Source: three-view drawing plus pictorial views. Frame: mm from the lowest corner of the part. Give positions to 0.01 mm unless a question says otherwise; leave off trailing zeros. Order: outer loops, then holes, each group sorted by start corner. A loop starts at its lowest first (then second) coordinate and runs counter-clockwise, first axis right, second up. Notation, with made-up numbers: (56, 33.5) -> (91, 33.5) arc R18 cw to (91, 62.5) -> close; hole circle Ø8 at (52, 39.25). An arc over 180 degrees is marked (long way). Answer in a Markdown table with one row per item.
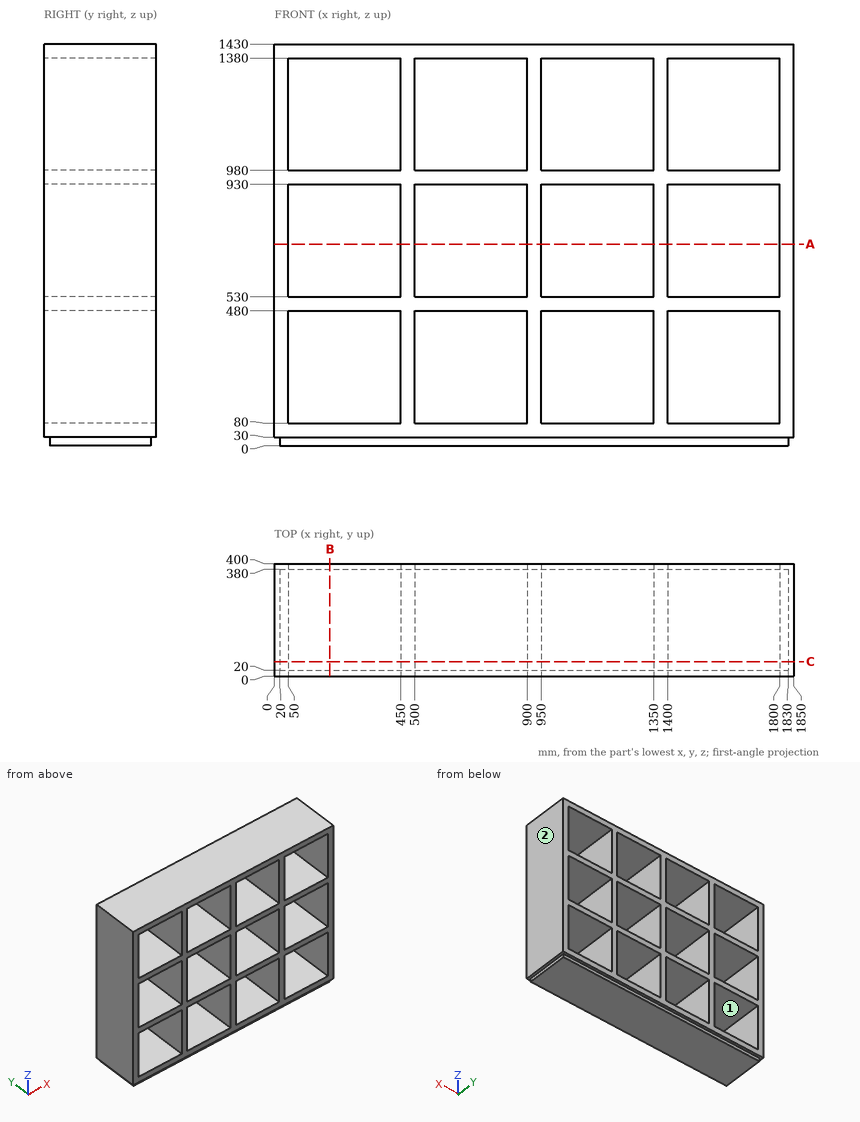
(1) Ray query, probe 1 along X at (y, z) = (269.5, 606); probe 2 along Z at (x, y) = (1578.5, 344). Return the intervals inside material, ascending.
A:
| item | result |
|---|---|
| probe 1 | x = 0 to 50, 450 to 500, 900 to 950, 1350 to 1400, 1800 to 1850 |
| probe 2 | z = 0 to 80, 480 to 530, 930 to 980, 1380 to 1430 |
(2) Section query A-A (z = 717.5). Return the cut outline in (x, y).
A:
| item | result |
|---|---|
| outline | (0, 0) -> (50, 0) -> (50, 400) -> (0, 400) -> close; (450, 0) -> (500, 0) -> (500, 400) -> (450, 400) -> close; (900, 0) -> (950, 0) -> (950, 400) -> (900, 400) -> close; (1350, 0) -> (1400, 0) -> (1400, 400) -> (1350, 400) -> close; (1800, 0) -> (1850, 0) -> (1850, 400) -> (1800, 400) -> close |
(3) Section query B-B (x = 198). Return the cut outline in (y, z).
A:
| item | result |
|---|---|
| outline | (0, 30) -> (20, 30) -> (20, 0) -> (380, 0) -> (380, 30) -> (400, 30) -> (400, 80) -> (0, 80) -> close; (0, 480) -> (400, 480) -> (400, 530) -> (0, 530) -> close; (0, 930) -> (400, 930) -> (400, 980) -> (0, 980) -> close; (0, 1380) -> (400, 1380) -> (400, 1430) -> (0, 1430) -> close |
(4) Pull-direction query (X, two-part tool) for the marked faces 1 and 2; classes: +X half, -X half, draft (parallel to the pull), parting line (faces both ways), or undercut.
A:
| item | result |
|---|---|
| face 1 | undercut |
| face 2 | +X half |
(5) Section query C-C (y = 51). Give the number of separate pieces and of enclosed holes in the cut face, plus the area to 3 significant figures.
A:
| item | result |
|---|---|
| separate pieces | 1 |
| enclosed holes | 12 |
| area | 724,000 mm^2 |
